Could you check a few things on this model? Use its own coordinates, in mm. A direction names the side the tool comes from. Give positions to 0.01 mm unless a question says otherwise; leave off trailing zeros. Order: outer loops, then holes, each group sorted by start corner. A loop starts at its lowest first (then second) coordinate and runs counter-clockwise, first axis right, second up.
(1) Imagine slicing it at A-A, the plane x = 66. Write out the boundary of the cut face in (y, z), then the cut area to 3 significant figures.
(2) If I drill on probe 1 along Y at (x, z) = (-75.5, 0.6); probe 2 along Y at (x, z) = (55, 0.45); probe 3 along Y at (x, z) = (27, 0.45), over which ranges is the centre line in solid material (lowest first)?
(3) On a 3-axis mill with a long thin cutter (end or side, diameter ignored), from which of +Z, -Z, +X, -X, +Y, -Y can I reach the whole of each face in a straight line? I mean faces 3 (the flat face through (-1, 0, 0)), 4 (the flat face through (10.94, -11.22, 0.99)). Say none if no direction works.
(4) Imagine slicing it at D-D, the plane x = -28. Write out the boundary of the cut face in (y, z), then the cut area to 3 significant figures.
(5) If we mould it in two halves opening along X, with no side actions, what happens to faces 1 (the flat face through (43.57, 11.3, 0.99)), 2 (the flat face through (-1, 0, 2))? For each: released by +X, released by -X, zero draft, split by the parting line, or undercut.
(6) Imagine slicing it at B-B, the plane x = 28.5. Write out the boundary of the cut face in (y, z).
(7) Imagine slicing it at C-C, the plane z = 0.35. State how many separate pieces and enclosed holes the cut face has, then the cut area to 3 significant figures.
from build123d import *

# Parameters (mm, degrees)
F1_W     = 180
F1_H     = 60
F1_W_2   = 5.451307
F1_H_2   = 16.88455
F1_W_3   = 5.450975
F1_W_4   = 27.255869
F1_H_3   = 5.628183
F2_DEPTH = 2
F3_SIZE  = 1


with BuildPart() as f2:
    # F1 (on Top) → F2 (new body)
    with BuildSketch(Plane.XY):
        Rectangle(F1_W, F1_H)
        Polygon((-40.883972, -14.070458), (-46.335113, -14.070458), (-46.335113, 2.814092), (-19.079077, 2.814092), (-19.079077, -14.070458), (-24.530383, -14.070458), (-24.530383, -2.814092), (-40.883972, -2.814092), align=None, mode=Mode.SUBTRACT)
        Polygon((5.451141, -8.442275), (8.17696, -5.628183), (8.17696, 2.814092), (13.627935, 2.814092), (13.627935, -8.442275), (8.17696, -14.070458), (-8.176628, -14.070458), (-13.627936, -8.442275), (-13.627936, 2.814092), (-8.176628, 2.814092), (-8.176628, -5.628183), (-5.451141, -8.442275), align=None, mode=Mode.SUBTRACT)
        with Locations((21.804896, -5.628183)):
            Rectangle(F1_W_2, F1_H_2, mode=Mode.SUBTRACT)
        with Locations((43.609624, -5.628183)):
            Rectangle(F1_W_3, F1_H_2, mode=Mode.SUBTRACT)
        Polygon((62.688701, 2.814092), (68.140008, 2.814092), (68.140008, -8.442275), (79.042289, -8.442275), (79.042289, -14.070458), (51.78642, -14.070458), (51.78642, -8.442275), (62.688701, -8.442275), align=None, mode=Mode.SUBTRACT)
        Polygon((-79.04229, 8.442275), (-79.04229, 14.070458), (-57.23756, 14.070458), (-51.786254, 8.442275), (-51.786254, 2.814092), (-57.23756, -2.814092), (-51.786254, -14.070458), (-57.23756, -14.070458), (-62.688701, -2.814092), (-73.591149, -2.814092), (-73.591149, -14.070458), (-79.04229, -14.070458), (-79.04229, 2.814092), (-59.963048, 2.814092), (-57.23756, 5.628183), (-59.963048, 8.442275), align=None, mode=Mode.SUBTRACT)
        Polygon((-46.335113, 8.442275), (-40.883972, 14.070458), (-24.530383, 14.070458), (-19.079077, 8.442275), align=None, mode=Mode.SUBTRACT)
        Polygon((-13.627936, 8.442275), (-8.176628, 14.070458), (8.17696, 14.070458), (13.627935, 8.442275), align=None, mode=Mode.SUBTRACT)
        Polygon((19.079242, 8.442275), (24.530549, 14.070458), (40.884137, 14.070458), (46.335112, 8.442275), align=None, mode=Mode.SUBTRACT)
        with Locations((65.414355, 11.256366)):
            Rectangle(F1_W_4, F1_H_3, mode=Mode.SUBTRACT)
    extrude(amount=F2_DEPTH)

    # F3
    f3_edges = [f2.edges().sort_by_distance(p)[0] for p in [
        (0, 30, 2),
        (0, -30, 2),
        (90, 0, 2),
        (-90, 0, 2),
    ]]
    chamfer(f3_edges, length=F3_SIZE)


solid = f2.part
Answer block:
1. outline: (-30, 0) - (-14.07, 0) - (-14.07, 2) - (-29, 2) - (-30, 1) - close; (2.81, 0) - (8.44, 0) - (8.44, 2) - (2.81, 2) - close; (14.07, 0) - (30, 0) - (30, 1) - (29, 2) - (14.07, 2) - close
1. area: 74.0 mm2
2. probe 1: y = -30 to -14.07, 2.81 to 8.44, 14.07 to 30
2. probe 2: y = -30 to -14.07, -8.44 to 8.44, 14.07 to 30
2. probe 3: y = -30 to 8.44, 14.07 to 30
3. face 3: -Z, +X, -X, +Y, -Y
3. face 4: +Z, -Z
4. outline: (-30, 0) - (-2.81, 0) - (-2.81, 2) - (-29, 2) - (-30, 1) - close; (2.81, 0) - (8.44, 0) - (8.44, 2) - (2.81, 2) - close; (14.07, 0) - (30, 0) - (30, 1) - (29, 2) - (14.07, 2) - close
4. area: 96.5 mm2
5. face 1: undercut
5. face 2: zero draft
6. outline: (-30, 0) - (8.44, 0) - (8.44, 2) - (-29, 2) - (-30, 1) - close; (14.07, 0) - (30, 0) - (30, 1) - (29, 2) - (14.07, 2) - close
7. separate pieces: 1
7. enclosed holes: 10
7. area: 8,910 mm2
